Geometry: see drawing. Coordinates: mm, zero at the bounding-box minimum. A direction names the side the tool comes from. Coordinates: 2 decimals unless noted, no trailing zeros. Order: outer loops, then holes, each group sorted by start corner. A loop starts at its lowest first (then second) coordinate and runs counter-clockwise, first axis right, second up. Notation, with made-up numbers: (19.5, 80) -> (53.5, 80) arc R26 cw to (53.5, 97) -> close; hole circle Ø3 at (-35, -32). An arc over 180 degrees is marked (long way). Write each question's results on one line, items separated by ' | '.
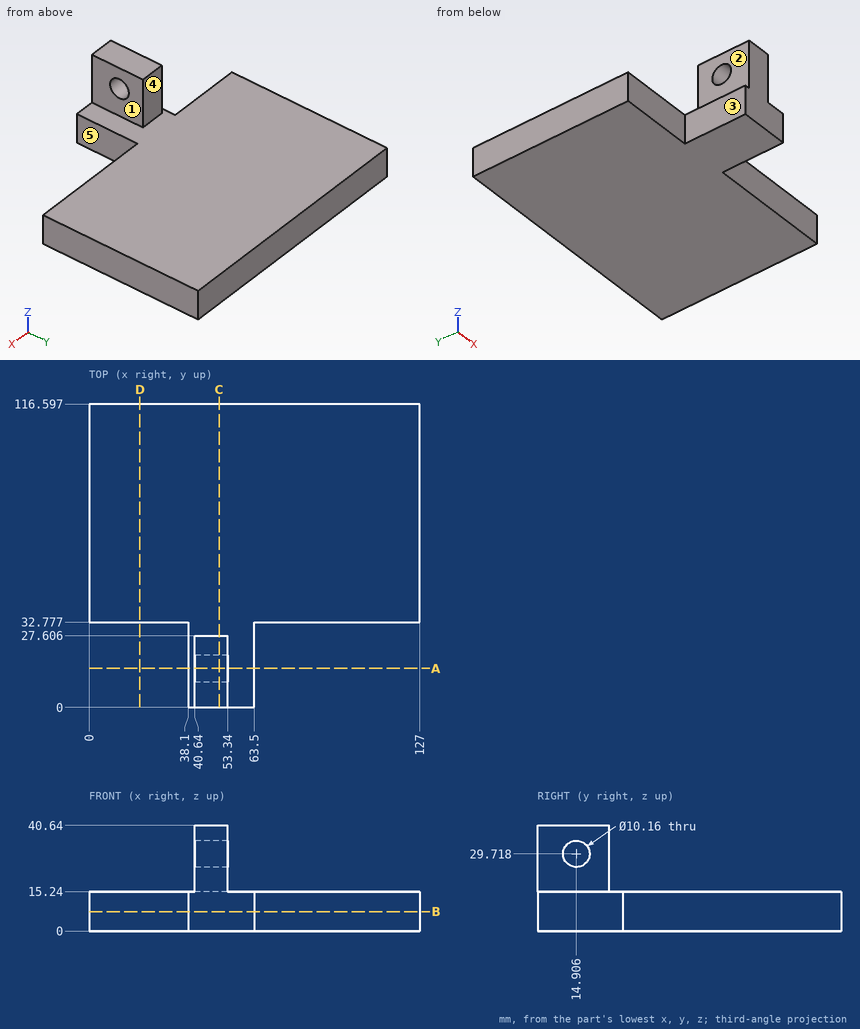
(1) Cut plane B-B, the plane z = 7.5. Return loops of the section in (x, y), plus the area to 3 significant figures.
Return value:
outline: (0, 32.78) -> (38.1, 32.78) -> (38.1, 0) -> (63.5, 0) -> (63.5, 32.78) -> (127, 32.78) -> (127, 116.6) -> (0, 116.6) -> close | area: 11,500 mm2
(2) Pin query (flat end, axial travel): P1, Ø12, axis at y = 23.5, z = 31, coming from the -X side; P2, Ø7.5, axis at x = 107, z = 4, coming from the -Y side; P3, Ø4.5, axis at y = 16.5, z = 7.5, coming from the -X side. Return the tip coordinate at first contact, or that it passes through.
Return value:
P1: x = 40.64 | P2: y = 32.78 | P3: x = 38.1
(3) Line query: line 1 along Z through (x, y) = (26, 99); line 2 along Y through (x, z) = (71, 9); line 3 along Y through (x, z) = (49, 27) (1 decimal). Output: solid intervals per line, ascending. Write a range as from..to.
Return value:
line 1: 0..15.24 | line 2: 32.78..116.6 | line 3: 0..10.6, 19.2..27.6
(4) Cut plane D-D, the plane x = 19.5. Return loops of the section in (y, z).
Return value:
outline: (32.78, 0) -> (116.6, 0) -> (116.6, 15.24) -> (32.78, 15.24) -> close
(5) Cut plane A-A, the plane y = 15. Return loops of the section in (x, z).
Return value:
outline: (38.1, 0) -> (63.5, 0) -> (63.5, 15.24) -> (53.34, 15.24) -> (53.34, 24.64) -> (40.64, 24.64) -> (40.64, 15.24) -> (38.1, 15.24) -> close; (40.64, 34.8) -> (53.34, 34.8) -> (53.34, 40.64) -> (40.64, 40.64) -> close
(6) Reachability of the marked faces 1, 2, 3, 4 and 5 from +Z, -Z, +X, -X, +Y, -Y: full face, straight path, thin tool, end or side. Return the list, or none.
Return value:
face 1: +Z, +X, +Y, -Y | face 2: +Z, -X, +Y, -Y | face 3: +Z, -Z, -X, -Y | face 4: +Z, +X, -X, +Y | face 5: +Z, -Z, +X, -Y
(7) Cut plane C-C, the plane x = 50. Return loops of the section in (y, z).
Return value:
outline: (0, 0) -> (116.6, 0) -> (116.6, 15.24) -> (27.61, 15.24) -> (27.61, 40.64) -> (0, 40.64) -> close; hole circle Ø10.16 at (14.91, 29.72)
